Input: part model. Units: mm. Frame: model coordinates. A direction names the side the tool comes from. Round coordinates to 2 decimals unless told otherwise and drop trailing zeros. Loops run counter-clockwise (first coordinate to the right, second up) from the corner with the lowest first, then second, coordinate; pieces in that order, holes last.
1) Ray query, line 1 along X through (y, z) = (2.5, 36); line 2 along Z through (x, y) = (11, 5.5); line 3 along Y through (x, z) = (18, 47). Return the intervals inside material, ascending.
2) Section D-D, the plane z = 15. Return loops of the section in (x, y).
3) First-contact query: pin 1 (1 mm diameter, centred on y = -6.5, z = 11.5, fed in from +X); pin 2 (12 mm diameter, centred on x = -2.5, y = 8, fed in from +Z); pin 3 (1.5 mm diameter, centred on x = -17, z = 7, fed in from +Y). Flat tips, straight axial feed; report the tip coordinate or a pass-through.
4) Section A-A, the plane y = 0. Return loops of the section in (x, z).
5) Section C-C, the plane z = 33. Return loops of the section in (x, y).
6) Access query for faces 1 (the face through (0, 0, 0)), 2 (the face through (6.7, -29.5, 50)), 3 (the face through (-2.708, 20.623, -0.789)). Directions: +Z, -Z, +X, -X, +Y, -Y. A direction counts if a zero-diameter tool reaches every point of the face in a straight line with its end or side. Return the directions, or none.
7) Draft query along X for faces 4 (the face through (-5.37, -24.17, 19.79)), 5 (the face through (22.13, -9.18, 19.79)), 6 (the face through (0, 0, -1.6)). Return one class per face: pulls with the +X half, pulls with the -X half, needs draft (parallel to the pull), parting line crosses it, or undercut.
from build123d import *

# Parameters (mm, degrees)
SKETCH_R      = 20.8
EXTRUDE_DEPTH = 1.6


with BuildPart() as cone001:
    # Cone001 → Cone001 (revolve)
    with BuildSketch(Plane.XZ):
        Polygon((0, 0), (20, 0), (30, 50), (0, 50), align=None)
    revolve(axis=Axis((0, 0, 0), (0, 0, 1)))


with BuildPart() as cut:
    # Cone → Cone (revolve)
    with BuildSketch(Plane.XZ):
        Polygon((0, 0), (20.8, 0), (30.8, 50), (0, 50), align=None)
    revolve(axis=Axis((0, 0, 0), (0, 0, 1)))

    # Cut: cut Cone001
    add(cone001.part, mode=Mode.SUBTRACT)


with BuildPart() as fusion:
    # Sketch → Extrude (new body)
    with BuildSketch(Plane.XY):
        Circle(SKETCH_R)
    extrude(amount=-EXTRUDE_DEPTH)

    # Fusion: union Cut
    add(cut.part)


solid = fusion.part
Final values:
1. line 1: x = -27.89 to -27.08, 27.08 to 27.89
1. line 2: z = -1.6 to 0
1. line 3: y = -24.25 to -23.25, 23.25 to 24.25
2. outline: circle Ø47.6 at (0, 0); hole circle Ø46 at (0, 0)
3. pin 1: stops at x = 22.34
3. pin 2: stops at z = 0
3. pin 3: stops at y = 15.15
4. outline: (-30.8, 50) - (-20.8, 0) - (-20.8, -1.6) - (20.8, -1.6) - (20.8, 0) - (30.8, 50) - (30, 50) - (20, 0) - (-20, 0) - (-30, 50) - close
5. outline: circle Ø54.8 at (0, 0); hole circle Ø53.2 at (0, 0)
6. face 1: +Z
6. face 2: +Z, +X, -X, +Y, -Y
6. face 3: -Z
7. face 4: parting line crosses it
7. face 5: undercut
7. face 6: needs draft
